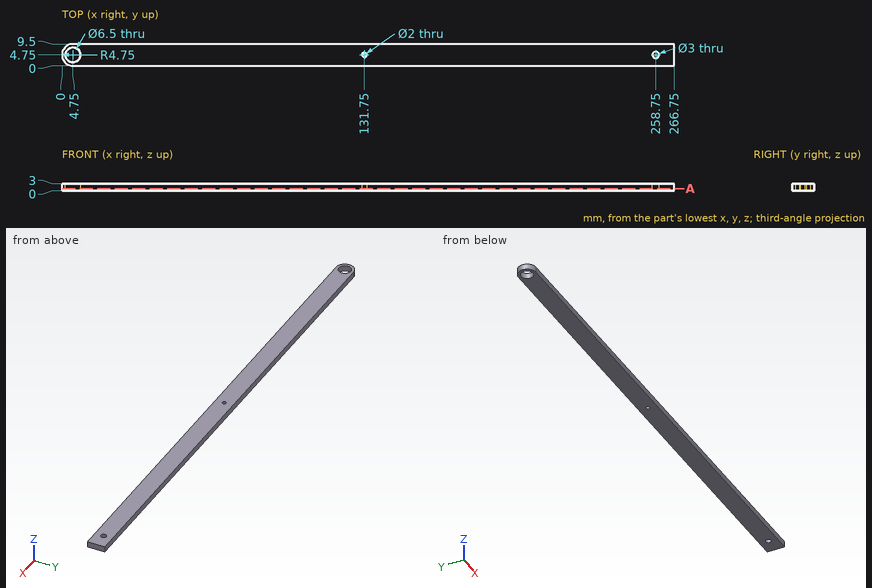
Study the drawing (mm; zero at the part's minimum x, y, z) and answer. Round coordinates to 2 decimals unless told otherwise and drop trailing zeros. Loops run counter-clockwise (first coordinate to the right, second up) from the corner with the lowest first, then second, coordinate; pieces in that order, holes last.
Q1. Given pin 1 Ø5 at (x, y) = (69.5, 3) entering from -Z, flat-ended and moving along its own axis, determine where the tip first touches the part or whether it passes through.
Q2. Find the intervals of material crossed by line 1 (X direction, y = 4, z = 0.2); line 2 (Y direction, x = 4.75, z = 2.1); line 3 (Y direction, x = 258.75, z = 0.95), in increasing order.
Q3. Section A-A, the plane z = 0.85 is taken. Determine the outline of the cut face in (x, y), then the cut area to 3 significant figures.
Completed:
1. pin 1: stops at z = 0
2. line 1: x = 0.06 to 1.59, 7.91 to 131.09, 132.41 to 257.45, 260.05 to 266.75
2. line 2: y = 0 to 1.5, 8 to 9.5
2. line 3: y = 0 to 3.25, 6.25 to 9.5
3. outline: (4.75, 0) - (266.75, 0) - (266.75, 9.5) - (4.75, 9.5) arc R4.75 ccw to start; hole circle Ø6.5 at (4.75, 4.75); hole circle Ø2 at (131.75, 4.75); hole circle Ø3 at (258.75, 4.75)
3. area: 2,480 mm2
